Verification items for this drawing (mm, ordinates from the low corner). Round coordinates to 2 decimals unless told otherwise and drop trailing zeros. Loops run counter-clockwise (first coordinate to the right, second up) from the corner with the lowest first, then second, coordinate; pieces in that order, holes last. Notation, with made-up numbers: (34.5, 73) - (91.5, 73) arc R29 cw to (91.5, 95) - close; hole circle Ø8 at (36.25, 75). An arc over 180 degrees is marked (long way). Use a Markdown table: item, result. Add a question column.
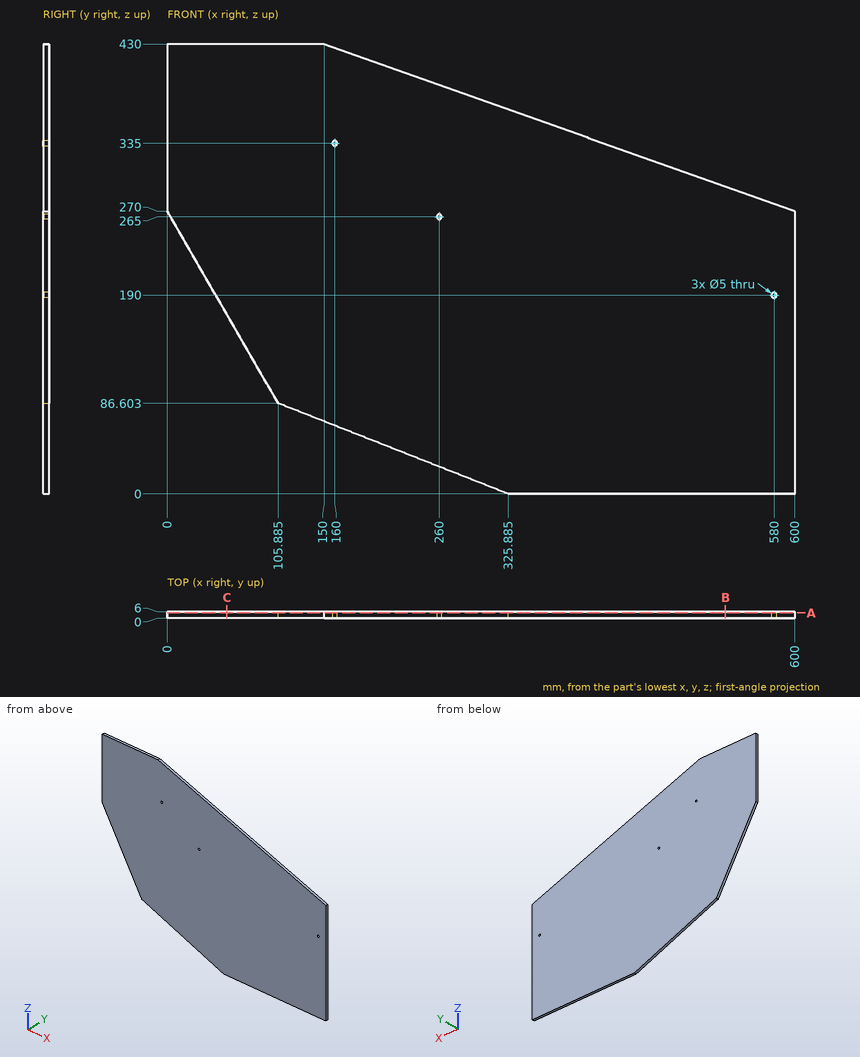
Q1. Section check B-B on x = 533.5. Record the cut outline in (y, z) (1 decimal), plus the area to 3 significant figures.
Q2. Thickness scan on line 1 along X through (y, z) = (2.2, 190); line 2 along Z through (x, y) = (260, 4.25) (1 decimal); line 3 along Z through (x, y) = (63, 4.9). Record the ranges inside material, lowest first.
Q3. Section check A-A on y = 5.1. Record the cut outline in (x, z) (1 decimal).
Q4. Section check C-C on x = 57. Record the cut outline in (y, z).
Q5. Go/stop test with a flat-tipped pin: pin 1 Ø1.5 at (y, z) = (5.5, 118.5) entering from -X (1 decimal). Record where the tip stops, or that it passes through.
Determined:
| question | item | result |
|---|---|---|
| 1 | outline | (0, 0) - (6, 0) - (6, 293.6) - (0, 293.6) - close |
| 1 | area | 1,760 mm² |
| 2 | line 1 | x = 46.19 to 577.5, 582.5 to 600 |
| 2 | line 2 | z = 25.9 to 262.5, 267.5 to 390.9 |
| 2 | line 3 | z = 160.88 to 430 |
| 3 | outline | (0, 270) - (105.9, 86.6) - (325.9, 0) - (600, 0) - (600, 270) - (150, 430) - (0, 430) - close; hole circle Ø5 at (160, 335); hole circle Ø5 at (260, 265); hole circle Ø5 at (580, 190) |
| 4 | outline | (0, 171.27) - (6, 171.27) - (6, 430) - (0, 430) - close |
| 5 | pin 1 | stops at x = 87 |
